Geometry: final body of the model. Coordinates: model frame, mm. A direction names the side the tool comes from. Give positions to 0.01 mm unless a question says otherwise; leave off trailing zeros. Write each loop counter-clockwise with the first axis right and the second up, starting at its lowest first coordinate (ties: lowest second). Pieces come first, ordered by that corner, then holes.
from build123d import *

# Parameters (mm, degrees)
SZKIC1_R                       = 14.5
SZKIC1_R_2                     = 5
DODANIE_WYCI_GNI_CIE1_DEPTH    = 15
M6_TAPPED_HOLE1_D              = 5
DODANIE_WYCI_GNI_CIE3_START    = -25
DODANIE_WYCI_GNI_CIE3_DEPTH    = 25
OTW_R_GWINTOWANY_M8X1_01_D     = 7
OTW_R_GWINTOWANY_M8X1_01_DEPTH = 18.896987833
OTW_R_GWINTOWANY_M8X1_01_TIP   = 2.103012167
WYTNIJ_WYCI_GNI_CIE2_DEPTH     = 10
WYTNIJ_WYCI_GNI_CIE4_DEPTH     = 20
SFAZOWANIE4_SIZE               = 10
WYTNIJ_WYCI_GNI_CIE5_DEPTH     = 5
SZKIC17_5_R                    = 7.5
WYTNIJ_WYCI_GNI_CIE6_DEPTH     = 163.311542951


with BuildPart() as part:
    # Szkic1 → Dodanie-wyciągnięcie1 (new, symmetric)
    with BuildSketch(Plane(origin=(0, 0, 0), x_dir=(0, 0, -1), z_dir=(1, 0, 0))):
        with BuildLine():
            Line((62.076569761, 109.385977671), (65.40069858, 86.060032436))
            ThreePointArc((65.40069858, 86.060032436), (67.080888035, 80.867469231), (70.408575711, 76.541704099))
            ThreePointArc((70.408575711, 76.541704099), (81.115709466, 65.086416999), (89.978943384, 52.151603499))
            ThreePointArc((89.978943384, 52.151603499), (92.32041193, 40.919666146), (87.495806927, 30.50995538))
            ThreePointArc((87.495806927, 30.50995538), (75.419960244, 0), (87.495806927, -30.50995538))
            ThreePointArc((87.495806927, -30.50995538), (92.32041193, -40.919666146), (89.978943384, -52.151603499))
            ThreePointArc((89.978943384, -52.151603499), (77.589025222, -69.25274843), (62, -83.498502981))
            Line((62, -83.498502981), (62, -100))
            ThreePointArc((62, -100), (58.828108774, -114.988630917), (49.856267202, -127.407407407))
            ThreePointArc((49.856267202, -127.407407407), (46.738768646, -129.329364235), (43.138357147, -130))
            Line((43.138357147, -130), (25, -130))
            Line((25, -130), (-25, -130))
            Line((-25, -130), (-43.138357147, -130))
            ThreePointArc((-43.138357147, -130), (-46.738768646, -129.329364235), (-49.856267202, -127.407407407))
            ThreePointArc((-49.856267202, -127.407407407), (-58.828108774, -114.988630917), (-62, -100))
            Line((-62, -100), (-62, -83.498502981))
            ThreePointArc((-62, -83.498502981), (-77.589025222, -69.25274843), (-89.978943384, -52.151603499))
            ThreePointArc((-89.978943384, -52.151603499), (-92.32041193, -40.919666146), (-87.495806927, -30.50995538))
            ThreePointArc((-87.495806927, -30.50995538), (-75.419960244, 0), (-87.495806927, 30.50995538))
            ThreePointArc((-87.495806927, 30.50995538), (-92.32041193, 40.919666146), (-89.978943384, 52.151603499))
            ThreePointArc((-89.978943384, 52.151603499), (-81.115709466, 65.086416999), (-70.408575711, 76.541704099))
            ThreePointArc((-70.408575711, 76.541704099), (-67.080888035, 80.867469231), (-65.40069858, 86.060032436))
            Line((-65.40069858, 86.060032436), (-62.076569761, 109.385977671))
            ThreePointArc((-62.076569761, 109.385977671), (-54.044566654, 124.12820267), (-38.316621209, 130))
            Line((-38.316621209, 130), (38.316621209, 130))
            ThreePointArc((38.316621209, 130), (54.044566654, 124.12820267), (62.076569761, 109.385977671))
        make_face()
        Circle(SZKIC1_R, mode=Mode.SUBTRACT)
        with Locations((-74.189369185, 43)):
            Circle(SZKIC1_R_2, mode=Mode.SUBTRACT)
        with Locations((-74.189369185, -43)):
            Circle(SZKIC1_R_2, mode=Mode.SUBTRACT)
        with BuildLine():
            Line((-25, -84), (25, -84))
            ThreePointArc((25, -84), (41, -100), (25, -116))
            Line((25, -116), (-25, -116))
            ThreePointArc((-25, -116), (-41, -100), (-25, -84))
        make_face(mode=Mode.SUBTRACT)
    extrude(amount=DODANIE_WYCI_GNI_CIE1_DEPTH, both=True)

    # M6 Tapped Hole1 (through all)
    with Locations(Plane(origin=(15, 0, 0), x_dir=(0, 0, -1), z_dir=(1, 0, 0))):
        with Locations((-50.510423527, 100), (29.489576473, 100)):
            Hole(M6_TAPPED_HOLE1_D / 2)

    # Szkic5 → Dodanie-wyciągnięcie3 (add)
    with BuildSketch(Plane.ZY.offset(-15).offset(DODANIE_WYCI_GNI_CIE3_START)):
        with BuildLine():
            Line((75.419960244, 0), (44.419960244, 0))
            Line((44.419960244, 0), (40.419960244, -4))
            Line((40.419960244, -4), (40.419960244, -6))
            Line((40.419960244, -6), (44.419960244, -10))
            Line((44.419960244, -10), (76.556013712, -10))
            ThreePointArc((76.556013712, -10), (75.704884126, -5.032161998), (75.419960244, 0))
        make_face()
    extrude(amount=DODANIE_WYCI_GNI_CIE3_DEPTH)

    # Otwór gwintowany M8x1.01
    with Locations(Plane(origin=(0, 0, 0), x_dir=(1, 0, 0), z_dir=(0, 1, 0))):
        with Locations((27.5, -60.419960244)):
            Hole(OTW_R_GWINTOWANY_M8X1_01_D / 2, depth=OTW_R_GWINTOWANY_M8X1_01_DEPTH)
            with Locations((0, 0, -(OTW_R_GWINTOWANY_M8X1_01_DEPTH + OTW_R_GWINTOWANY_M8X1_01_TIP / 2))):  # 118° drill point
                Cone(0, OTW_R_GWINTOWANY_M8X1_01_D / 2, OTW_R_GWINTOWANY_M8X1_01_TIP, mode=Mode.SUBTRACT)

    # Szkic12 → Wytnij-wyciągnięcie2 (cut)
    with BuildSketch(Plane(origin=(15, 0, 0), x_dir=(0, 0, -1), z_dir=(1, 0, 0))):
        with BuildLine():
            Line((9.489576473, 105), (-30.510423527, 105))
            ThreePointArc((-30.510423527, 105), (-35.510423527, 100), (-30.510423527, 95))
            Line((-30.510423527, 95), (9.489576473, 95))
            ThreePointArc((9.489576473, 95), (14.489576473, 100), (9.489576473, 105))
        make_face()
    extrude(amount=-WYTNIJ_WYCI_GNI_CIE2_DEPTH, mode=Mode.SUBTRACT)

    # Szkic16 → Wytnij-wyciągnięcie4 (cut)
    with BuildSketch(Plane(origin=(15, 0, 0), x_dir=(0, 0, -1), z_dir=(1, 0, 0))):
        with BuildLine():
            Line((-43.138357147, -130), (43.138357147, -130))
            ThreePointArc((43.138357147, -130), (46.738768646, -129.329364235), (49.856267202, -127.407407407))
            ThreePointArc((49.856267202, -127.407407407), (58.828108774, -114.988630917), (62, -100))
            Line((62, -100), (62, -83.498502981))
            ThreePointArc((62, -83.498502981), (69.784912958, -77.110738056), (76.915538092, -70))
            Line((76.915538092, -70), (-76.915538092, -70))
            ThreePointArc((-76.915538092, -70), (-69.784912958, -77.110738056), (-62, -83.498502981))
            Line((-62, -83.498502981), (-62, -100))
            ThreePointArc((-62, -100), (-58.828108774, -114.988630917), (-49.856267202, -127.407407407))
            ThreePointArc((-49.856267202, -127.407407407), (-46.738768646, -129.329364235), (-43.138357147, -130))
        make_face()
        with BuildLine():
            Line((-25, -116), (25, -116))
            ThreePointArc((25, -116), (41, -100), (25, -84))
            Line((25, -84), (-25, -84))
            ThreePointArc((-25, -84), (-41, -100), (-25, -116))
        make_face(mode=Mode.SUBTRACT)
    extrude(amount=-WYTNIJ_WYCI_GNI_CIE4_DEPTH, mode=Mode.SUBTRACT)

    # Sfazowanie4
    sfazowanie4_edges = [part.edges().sort_by_distance(p)[0] for p in [
        (15, -70, 0),
    ]]
    chamfer(sfazowanie4_edges, length=SFAZOWANIE4_SIZE)

    # Szkic17 → Wytnij-wyciągnięcie5 (cut)
    with BuildSketch(Plane(origin=(15, 0, 0), x_dir=(0, 0, -1), z_dir=(1, 0, 0))):
        with BuildLine():
            Line((31.578571429, -10.936663671), (45.292857143, -8.957177034))
            ThreePointArc((45.292857143, -8.957177034), (53.05, 0), (45.292857142, 8.957177033))
            Line((45.292857142, 8.957177033), (31.578571428, 10.93666367))
            ThreePointArc((31.578571428, 10.93666367), (22.462605729, 8.080234378), (18.98012619, -0.815402484))
            ThreePointArc((18.98012619, -0.815402484), (23.079412621, -8.614404816), (31.578571429, -10.936663671))
        make_face()
    extrude(amount=-WYTNIJ_WYCI_GNI_CIE5_DEPTH, mode=Mode.SUBTRACT)

    # Szkic17<5> → Wytnij-wyciągnięcie6 (cut, through all)
    with BuildSketch(Plane(origin=(15, 0, 0), x_dir=(0, 0, -1), z_dir=(1, 0, 0))):
        with Locations((30, -1e-09)):
            Circle(SZKIC17_5_R)
    extrude(amount=-WYTNIJ_WYCI_GNI_CIE6_DEPTH, mode=Mode.SUBTRACT)


solid = part.part
Q1. Pin query (flat end, axial travel): P1, Ø1, axis at x = 10, y = 39.5, coming from the -Z side; P2, Ø24.5, axis at y = 4, z = -33.5, coming from the +X side; P3, Ø3, axis at x = -8, y = -94, coming from the +Z side. Return the tip coordinate at first contact, or that it passes through.
Filled sheet:
P1: stops at z = -92.19
P2: stops at x = 15
P3: stops at z = 62
Q2. Section B-B on y = -43. Output: boundary loops of the cut face in (x, z), plus the area to 3 significant figures.
Filled sheet:
outline: (-15, -92.44) - (15, -92.44) - (15, 69.19) - (-15, 69.19) - close; (-15, 79.19) - (15, 79.19) - (15, 92.44) - (-15, 92.44) - close
area: 5,250 mm2
Q3. Access query for faces 1 (the cylindrical face through (-10, -100, -41)), 2 (the flat face through (0, -70, -1)), 3 (the flat face through (-10, -92, -62)), 4 (the cylindrical face through (10.07, 99.89, -14.49)). Directions: +Z, -Z, +X, -X, +Y, -Y. A direction counts if a zero-diameter tool reaches every point of the face in a straight line with its end or side. Return the directions, or none.
Filled sheet:
face 1: +X, -X
face 2: +Z, -Z, +X, -Y
face 3: -Z, +X, -X, -Y
face 4: +X
Q4. Ray query, line 1 along Z through (x, y) = (5, 0.5); line 2 along Y through (x, z) = (-7, 21); line 3 along Y through (x, z) = (7.5, -8). Return the intervals inside material, ascending.
Filled sheet:
line 1: z = -75.42 to -37.48, -22.52 to -14.49, 14.49 to 75.42
line 2: y = -130 to -116, -84 to 130
line 3: y = -67.5 to -12.09, 12.09 to 95, 105 to 130
Q5. Pull-direction query (Z, two-part tool) for faces 5 (the cylindrical face through (0.21, 124.285, -53.862)), 6 (the cylindrical face through (-9.93, -129.35, 46.69)), 7 (the cylindrical face through (-10, -100, 41)); classes: released by +Z, released by -Z, zero draft, split by the parting line, or undercut.
Filled sheet:
face 5: released by -Z
face 6: released by +Z
face 7: undercut
Q6. Section D-D on x = 19.5. Output: boundary loops of the cut face in (y, z).
Filled sheet:
outline: (-10, 44.42) - (-6, 40.42) - (-4, 40.42) - (0, 44.42) - (0, 75.42) arc R44.58 cw to (-10, 76.56) - close
Q7. Section A-A on z = 0. Output: boundary loops of the cut face in (x, y).
Filled sheet:
outline: (-15, -130) - (-5, -130) - (-5, -116) - (-15, -116) - close; (-15, -84) - (-5, -84) - (-5, -70) - (5, -70) - (15, -60) - (15, -14.5) - (-15, -14.5) - close; (-15, 14.5) - (15, 14.5) - (15, 95) - (5, 95) - (5, 105) - (15, 105) - (15, 130) - (-15, 130) - close
Q8. Section C-C on x = -1. Output: boundary loops of the cut face in (y, z).
Filled sheet:
outline: (-70, -76.92) arc R104 ccw to (-52.15, -89.98) arc R18.25 ccw to (-30.51, -87.5) arc R44.58 cw to (30.51, -87.5) arc R18.25 ccw to (52.15, -89.98) arc R104 ccw to (76.54, -70.41) arc R16 cw to (86.06, -65.4) - (109.39, -62.08) arc R24 ccw to (130, -38.32) - (130, 38.32) arc R24 ccw to (109.39, 62.08) - (86.06, 65.4) arc R16 cw to (76.54, 70.41) arc R104 ccw to (52.15, 89.98) arc R18.25 ccw to (30.51, 87.5) arc R44.58 cw to (-30.51, 87.5) arc R18.25 ccw to (-52.15, 89.98) arc R104 ccw to (-70, 76.92) - close; hole circle Ø10 at (-43, 74.19); hole circle Ø29 at (0, 0); hole circle Ø15 at (0, -30); hole circle Ø10 at (43, 74.19); hole circle Ø5 at (100, -29.49); hole circle Ø5 at (100, 50.51)
